from build123d import *

# Parameters (mm, degrees)
EXTRUDE_1_DEPTH     = 5
SKETCH_2_R          = 1.25
CUT_EXTRUDE_1_DEPTH = 2.5
CUT_EXTRUDE_START   = -2.5
SKETCH_3_R          = 1.25
CUT_EXTRUDE_2_DEPTH = 2.5
CHAMFER_1_SIZE      = 0.25
FILLET_1_R          = 0.1


with BuildPart() as part:
    # Эскиз1 → Бобышка-Вытянуть1 (new body)
    with BuildSketch(Plane.XY):
        Polygon((2.886751346, 0), (1.443375673, 2.5), (-1.443375673, 2.5), (-2.886751346, 0), (-1.443375673, -2.5), (1.443375673, -2.5), align=None)
    extrude(amount=EXTRUDE_1_DEPTH)

    # Эскиз2 → Вырез-Вытянуть1 (cut)
    with BuildSketch(Plane.XY.offset(5)):
        Circle(SKETCH_2_R)
    extrude(amount=-CUT_EXTRUDE_1_DEPTH, mode=Mode.SUBTRACT)

    # Эскиз3 → Вырез-Вытянуть2 (cut)
    with BuildSketch(Plane(origin=(0, 0, 0), x_dir=(-1, 0, 0), z_dir=(0, 0, -1)).offset(CUT_EXTRUDE_START)):
        with Locations(Location((0, 0, 0), (0, 0, 180))):
            Circle(SKETCH_3_R)
    extrude(amount=CUT_EXTRUDE_2_DEPTH, mode=Mode.SUBTRACT)

    # Фаска1
    chamfer_1_edges = [part.edges().sort_by_distance(p)[0] for p in [
        (-1.25, 0, 5),
        (-1.25, 0, 0),
    ]]
    chamfer(chamfer_1_edges, length=CHAMFER_1_SIZE)

    # Скругление1
    fillet_1_edges = [part.edges().sort_by_distance(p)[0] for p in [
        (0, 2.5, 5),
        (1.443375673, -2.5, 2.5),
        (-1.443375673, -2.5, 2.5),
        (-2.886751346, 0, 2.5),
        (-1.443375673, 2.5, 2.5),
        (1.443375673, 2.5, 2.5),
        (2.886751346, 0, 2.5),
        (-2.165063509, 1.25, 5),
        (-2.165063509, -1.25, 5),
        (0, -2.5, 5),
        (2.165063509, -1.25, 5),
        (0, -2.5, 0),
        (-2.165063509, -1.25, 0),
        (-2.165063509, 1.25, 0),
        (2.165063509, 1.25, 5),
        (0, 2.5, 0),
        (2.165063509, 1.25, 0),
        (2.165063509, -1.25, 0),
    ]]
    fillet(fillet_1_edges, radius=FILLET_1_R)


solid = part.part
Input: part model. Units: mm. Frame: model coordinates. Round coordinates to 2 decimals unless told otherwise and drop trailing zeros. Loops run counter-clockwise (first coordinate to the right, second up) from the corner with the lowest first, then second, coordinate; pieces in that order, holes last. Notation, with made-up numbers: M 69,84.5 L 99,84.5 A35 ccw 99,119.5 Z; hole C 76,-21.75 d6. An arc over 180 degrees is marked long. Answer as CSV lines item,"result". Start each with the question number.
(1) Line query: line 1 (Y direction, x = 0, z = 3.6); line 2 (Z direction, x = 2.5, y = 0.5); line 3 (Y direction, x = 1.4, z = 3.15). Output: solid intervals per line, ascending. Write a range as [from, to].
(2) Section A-A, the plane x = 0. Output: boundary loops of the cut face in (y, z), plus the area to 3 significant figures.
(3) First-contact query: pin 1 (2 mm diameter, centred on x = -1.5, y = -2, fed in from -Z); pin 2 (1 mm diameter, centred on x = 2.5, z = 3.5, fed in from -Y). Flat tips, straight axial feed; report the tip coordinate or a pass-through.
(4) Section B-B, the plane z = 2.35. Output: boundary loops of the cut face in (x, y), plus the area to 3 significant figures.
Values found:
1,line 1,"y = [-2.5, -1.25], [1.25, 2.5]"
1,line 2,"z = [0, 5]"
1,line 3,"y = [-2.5, 2.5]"
2,outline,"M -2.5,0.1 A0.1 ccw -2.4,0 L -1.5,0 L -1.25,0.25 L -1.25,4.75 L -1.5,5 L -2.4,5 A0.1 ccw -2.5,4.9 Z; M 1.25,0.25 L 1.5,0 L 2.4,0 A0.1 ccw 2.5,0.1 L 2.5,4.9 A0.1 ccw 2.4,5 L 1.5,5 L 1.25,4.75 Z"
2,area,"12.4 mm²"
3,pin 1,"stops at z = 0"
3,pin 2,"stops at y = -1.54"
4,outline,"M -2.86,-0.05 L -1.47,-2.45 A0.1 ccw -1.39,-2.5 L 1.39,-2.5 A0.1 ccw 1.47,-2.45 L 2.86,-0.05 A0.1 ccw 2.86,0.05 L 1.47,2.45 A0.1 ccw 1.39,2.5 L -1.39,2.5 A0.1 ccw -1.47,2.45 L -2.86,0.05 A0.1 ccw Z; hole C 0,0 d2.5"
4,area,"16.7 mm²"
